```python
from build123d import *

# Parameters (mm, degrees)
F2_SIZE  = 1
F4_DEPTH = 10
F6_DEPTH = 6


with BuildPart() as f1:
    # F0 (on Front) → F1 (revolve)
    with BuildSketch(Plane.XZ):
        Polygon((0, 12.5), (0, 4), (30, 4), (30, 6), (12, 6), (12, 5.5), (10, 5.5), (10, 12.5), align=None)
    revolve(axis=Axis((7.8071541328, 0, 0), (1, 0, 0)))

    # F2
    f2_edges = [f1.edges().sort_by_distance(p)[0] for p in [
        (30, 0, -6),
        (10, 0, -12.5),
        (0, 0, -12.5),
    ]]
    chamfer(f2_edges, length=F2_SIZE)

    # F3 (on face) → F4 (cut)
    with BuildSketch(Plane(origin=(0, 0, 0), x_dir=(0, -1, 0), z_dir=(-1, 0, 0))):
        with BuildLine():
            ThreePointArc((3.2454993279, -12.0713186567), (8.0348451211, -9.575555539), (11.3243531583, -5.2923553873))
            ThreePointArc((11.3243531583, -5.2923553873), (6.106482292, -7.2774222096), (3.2454993279, -12.0713186567))
        make_face()
    extrude(amount=-F4_DEPTH, mode=Mode.SUBTRACT)

    # F5 (on face) → F6 (cut)
    with BuildSketch(Plane(origin=(0, 0, 0), x_dir=(0, -1, 0), z_dir=(-1, 0, 0))):
        with BuildLine():
            ThreePointArc((9.5, 0), (8.6099239768, -4.0148734865), (6.106482292, -7.2774222096))
            ThreePointArc((6.106482292, -7.2774222096), (8.003069241, -6.0735072132), (10.1488083402, -5.4084830844))
            ThreePointArc((10.1488083402, -5.4084830844), (10.7345609878, -5.3299734663), (11.3243531583, -5.2923553873))
            ThreePointArc((11.3243531583, -5.2923553873), (12.4999954848, -0.0106244522), (11.3333333333, 5.2730973399))
            ThreePointArc((11.3333333333, 5.2730973399), (9.9714052703, 2.7913557041), (9.5, 0))
        make_face()
    extrude(amount=-F6_DEPTH, mode=Mode.SUBTRACT)


solid = f1.part
```
Check sheet for the modelled part. Datum: model origin and axes. Units: mm. A direction names the side the tool comes from. Round coordinates to 2 decimals unless told otherwise and drop trailing zeros. Loops run counter-clockwise (first coordinate to the right, second up) from the corner with the lowest first, then second, coordinate; pieces in that order, holes last. Notation, with made-up numbers: (77, 42.25) - (116, 42.25) arc R16 ccw to (116, 61.25) - close; hole circle Ø2 at (-23.75, 57.5). An arc over 180 degrees is marked (long way). Write item = value, one per line. Start each with the question number.
Q1. Thickness scan on L1, parallel to Z at x = 12.5, y = 0; L2, parallel to Z at x = 11, y = 0. Record the ranges inside material, lowest first.
Q2. Access from +Z, -Z, +X, -X, +Y, -Y to the whole of each face (thin tool, end or side, straight path). Record for faces 1 (the face through (10.99, 5.37, -1.19)), 2 (the face through (20, 0, -6)), 3 (the face through (0.17, 10.73, 4.59)), 4 (the face through (2.958, -9.985, 2.829)), 5 (the face through (4.944, 8.392, 9.264)).
Q3. Depth check by flat-ended pin: P1, Ø8, axis at x = 23.5, y = -6.5, coming from the +Z side; P2, Ø6, axis at x = 10, z = -1, coming from the -Y side; P3, Ø1.5, axis at x = 3.5, z = 9.5, coming from the -Y side; P4, Ø8, axis at x = 12.5, y = 10, coming from the -Z side. Enter the tip coordinate at first touch or a pass-through.
Q4. Section check A-A (y = 0). Record the boundary of the cut face in (x, z).
Q5. Section check C-C (x = 18). Record the boundary of the cut face in (y, z), plus the area to 3 significant figures.
Q6. Section check B-B (x = 3.5). Record the boundary of the cut face in (y, z).
Q7. Release check for a two-part mould opening along Z. For faces 6 (the face through (0, 5, 0)), 7 (the face through (15.21, 3.905, -0.867)), 8 (the face through (6.041, -5.255, -8.099)) record: pulls with the +Z half, pulls with the -Z half, needs draft (parallel to the pull), parting line crosses it, or undercut.
Derived:
q1.L1 = -6 to -4, 4 to 6
q1.L2 = -5.5 to -4, 4 to 5.5
q2.face_1 = none
q2.face_2 = +X
q2.face_3 = -X
q2.face_4 = -Z, -X, -Y
q2.face_5 = +X, -X
q3.P1 = 5.45
q3.P2 = -12.5
q3.P3 = -8.93
q3.P4 = -9.56
q4.outline = (0, -11.5) - (1, -12.5) - (9, -12.5) - (10, -11.5) - (10, -5.5) - (12, -5.5) - (12, -6) - (29, -6) - (30, -5) - (30, -4) - (0, -4) - close; (0, 4) - (30, 4) - (30, 5) - (29, 6) - (12, 6) - (12, 5.5) - (10, 5.5) - (10, 11.5) - (9, 12.5) - (1, 12.5) - (0, 11.5) - close
q5.outline = circle Ø12 at (0, 0); hole circle Ø8 at (0, 0)
q5.area = 62.8 mm^2
q6.outline = (-11.33, 5.27) arc R8.5 cw to (-9.5, 0) arc R9.5 ccw to (-6.11, -7.28) arc R8.5 cw to (-3.25, -12.07) arc R12.5 ccw (long way) to start; hole circle Ø8 at (0, 0)
q7.face_6 = needs draft
q7.face_7 = undercut
q7.face_8 = pulls with the -Z half
